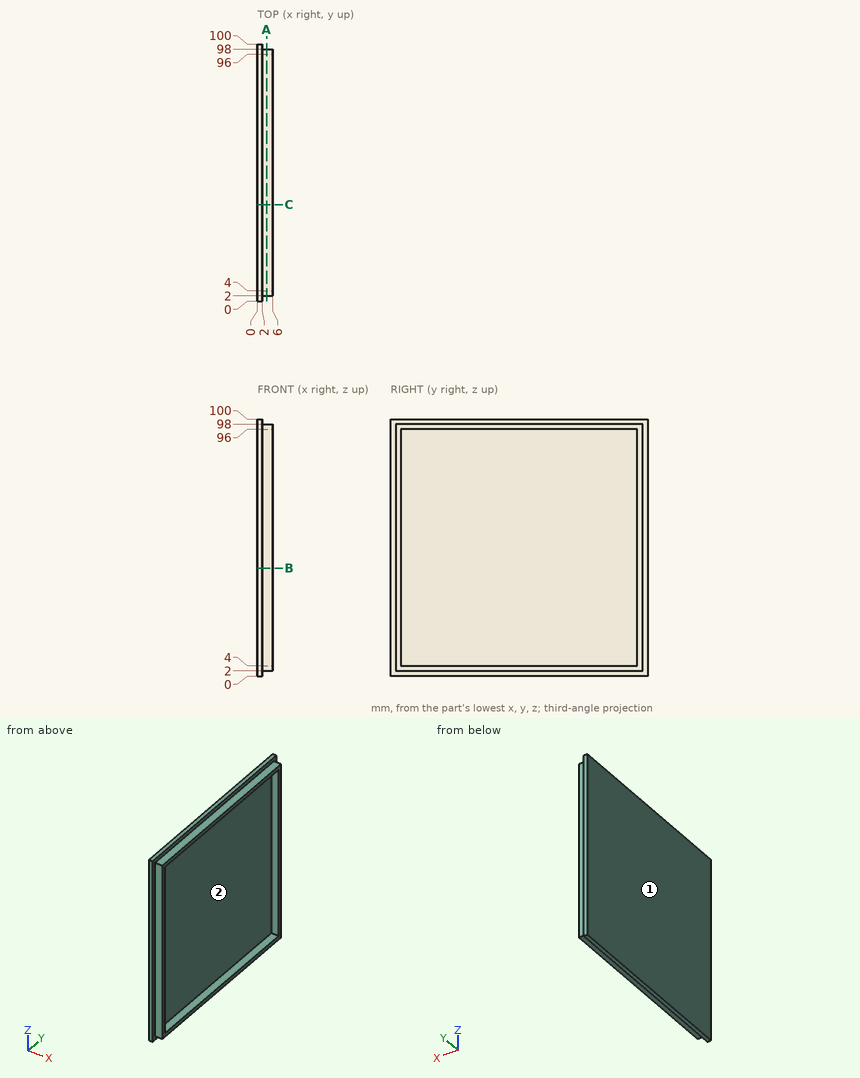
Here's the drawing with two shaded views (mm, measured from the low corner). I have some questions. A direction names the side the tool comes from. Give positions to 0.01 mm unless a question says otherwise; leave off trailing zeros. Order: outer loops, then holes, each group sorted by start corner. A loop starts at its lowest first (then second) coordinate and runs counter-clockwise, first axis right, second up. Notation, with made-up numbers: (74, -26.75) -> (98, -26.75) arc R19 ccw to (98, -11.75) -> close; hole circle Ø7 at (27.25, 26). An arc over 180 degrees is marked (long way). Use a Markdown table: item, result. Add a question column.
Item 1: Imagine slicing it at B-B on z = 42. Please give me the cut outline in (x, y).
Item 2: I need wall thicknesses on line 1 (Z direction, x = 3.5, y = 55.5); line 2 (X direction, y = 5.5, z = 27). Which ranges of each line are inside material? Lowest first, please.
Item 3: For the marked faces 1 and 2, which set-ups out of +Z, -Z, +X, -X, +Y, -Y let a thin tool reach every point of the face, with its end or its side?
Item 4: Will these pins go through, and if not, where does the flat tip stop? pin 1 (2 mm diameter, centred on x = 5, y = 52, fed in from +Z); pin 2 (2 mm diameter, centred on x = 5, z = 23, fed in from -Y); pin 3 (3 mm diameter, centred on x = 4.5, y = 50, fed in from -Z).
Item 5: Imagine slicing it at A-A on x = 3.6. Please give me the cut outline in (y, z).
Data:
| question | item | result |
|---|---|---|
| 1 | outline | (0, 0) -> (2, 0) -> (2, 2) -> (6, 2) -> (6, 4) -> (2, 4) -> (2, 96) -> (6, 96) -> (6, 98) -> (2, 98) -> (2, 100) -> (0, 100) -> close |
| 2 | line 1 | z = 2 to 4, 96 to 98 |
| 2 | line 2 | x = 0 to 2 |
| 3 | face 1 | +Z, -Z, -X, +Y, -Y |
| 3 | face 2 | +X |
| 4 | pin 1 | stops at z = 98 |
| 4 | pin 2 | stops at y = 2 |
| 4 | pin 3 | stops at z = 2 |
| 5 | outline | (2, 2) -> (98, 2) -> (98, 98) -> (2, 98) -> close; hole (4, 4) -> (96, 4) -> (96, 96) -> (4, 96) -> close |
